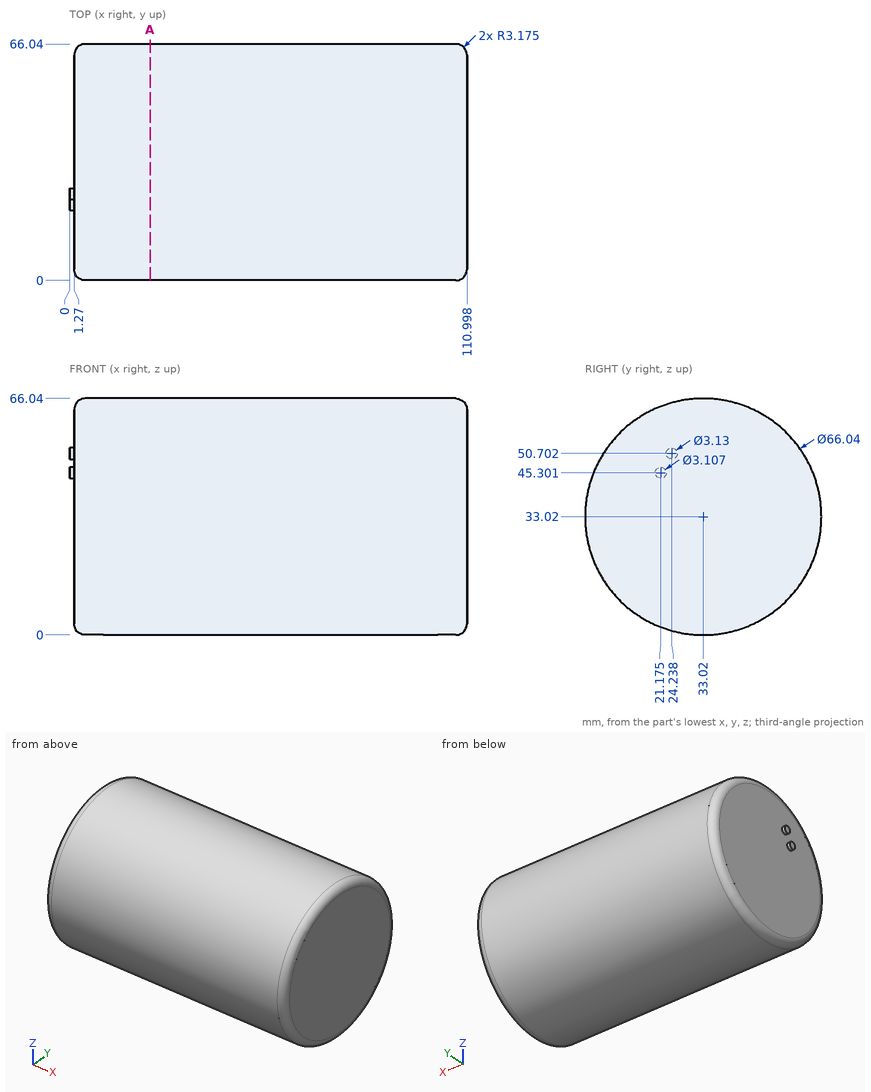
Source: three-view drawing plus pictorial views. Frame: mm from the lowest corner of the part. Give positions to 0.01 mm unless a question says otherwise; leave off trailing zeros. Order: outer loops, then holes, each group sorted by start corner. A loop starts at its lowest first (then second) coordinate and runs counter-clockwise, first axis right, second up. Notation, with made-up numbers: (-14.75, 36) -> (17.25, 36) arc R8 ccw to (17.25, 44) -> close; hole circle Ø4 at (-24.5, 37.25). An arc over 180 degrees is marked (long way). Write each question's results on one line, items separated by ' | '. Start each with the question number.
Item 1: Line query: line 1 (X direction, y = 8, z = 47); line 2 (Z direction, x = 84, y = 33.5); line 3 (Y direction, x = 103, z = 51) (1 decimal). Output: solid intervals per line, ascending.
Item 2: Cut plane A-A on x = 22.5. Return the cut outline in (y, z).
Item 3: Contact query for flat-ended pins moving along their axis: P1, Ø10, axis at x = 90, z = 24.5, coming from the -Y side; P2, Ø4, axis at x = 82.5, y = 50, coming from the -Z side; P3, Ø10, axis at x = 88, y = 39, coming from the -Z side (1 decimal). Output: stop coordinate, or through.
Established:
1) line 1: 1.27 to 111 | line 2: 0 to 66.04 | line 3: 5.3 to 60.7
2) outline: circle Ø66.04 at (33.02, 33.02)
3) P1: y = 0.19 | P2: z = 3.59 | P3: z = 0
